CAD build for the part. Positions are in the model's coordinates, mm. Face numbers are marked on the shaded views. Round coordinates to 2 decimals unless told otherwise and drop trailing zeros. Loops run counter-clockwise (first coordinate to the right, second up) from the corner with the lowest first, then second, coordinate; pieces in that order, holes last.
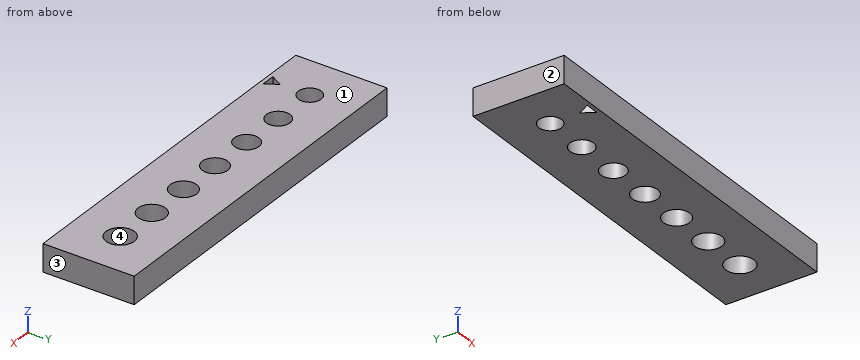
```python
from build123d import *

# Parameters (mm, degrees)
SKETCH_W   = 40
SKETCH_H   = 10
SKETCH_R   = 1.25
SKETCH_R_2 = 1.35
SKETCH_R_3 = 1.3
SKETCH_R_4 = 1.4
SKETCH_R_5 = 1.45
SKETCH_R_6 = 1.5
SKETCH_R_7 = 1.55
PAD_DEPTH  = 3


with BuildPart() as part:
    # Sketch → Pad (new body)
    with BuildSketch(Plane.XY):
        with Locations((20, 5)):
            Rectangle(SKETCH_W, SKETCH_H)
        with Locations((5, 5)):
            Circle(SKETCH_R, mode=Mode.SUBTRACT)
        with Locations((15, 5)):
            Circle(SKETCH_R_2, mode=Mode.SUBTRACT)
        with Locations((10, 5)):
            Circle(SKETCH_R_3, mode=Mode.SUBTRACT)
        with Locations((20, 5)):
            Circle(SKETCH_R_4, mode=Mode.SUBTRACT)
        with Locations((25, 5)):
            Circle(SKETCH_R_5, mode=Mode.SUBTRACT)
        with Locations((30, 5)):
            Circle(SKETCH_R_6, mode=Mode.SUBTRACT)
        with Locations((35, 5)):
            Circle(SKETCH_R_7, mode=Mode.SUBTRACT)
        Polygon((4.25, 0.433013), (5.75, 0.433013), (5, 1.732051), align=None, mode=Mode.SUBTRACT)
    extrude(amount=PAD_DEPTH)


solid = part.part
```
Item 1: Cut at B-B, the plane y = 5. State how many separate pieces and enclosed holes the cut face has, plus the area to 3 significant figures.
Answers follow:
separate pieces: 8
enclosed holes: 0
area: 61.2 mm2
Item 2: Two-plate mould, pull along X, no slides. Class the marked faces 1, 2, 3 and 4: released by +X, released by -X, zero draft, split by the parting line, or undercut.
Answers follow:
face 1: zero draft
face 2: released by -X
face 3: released by +X
face 4: undercut
Item 3: Cut at D-D, the plane x = 15. Give the cut face in (y, z), plus the area to 3 significant figures.
Answers follow:
outline: (0, 0) - (3.65, 0) - (3.65, 3) - (0, 3) - close; (6.35, 0) - (10, 0) - (10, 3) - (6.35, 3) - close
area: 21.9 mm2
Item 4: Cut at A-A, the plane x = 20. Give the cut face in (y, z), plus the area to 3 significant figures.
Answers follow:
outline: (0, 0) - (3.6, 0) - (3.6, 3) - (0, 3) - close; (6.4, 0) - (10, 0) - (10, 3) - (6.4, 3) - close
area: 21.6 mm2
Item 5: Flat gauge pin, fed straight in: P1, Ø6, axis at x = 30.5, y = 3.5, coming from the -Z side. Where does the tip first touch, or does it go through?
Answers follow:
P1: stops at z = 0
Item 6: Probe line 1 (Y direction, x = 10, z = 0.7); line 2 (Y direction, x = 30, z = 1.8); line 3 (X direction, y = 1, z = 0.6). List the from-to ranges inside material, lowest first.
Answers follow:
line 1: y = 0 to 3.7, 6.3 to 10
line 2: y = 0 to 3.5, 6.5 to 10
line 3: x = 0 to 4.58, 5.42 to 40
